from build123d import *

# Parameters (mm, degrees)
BOSS_EXTRUDE1_DEPTH      = 2
BOSS_EXTRUDE1_DEPTH_BACK = 0.2
SKETCH1_W                = 4.602701487
SKETCH1_H                = 5.995472756
SKETCH1_W_2              = 1.15
SKETCH1_H_2              = 4.4
BOSS_EXTRUDE2_REACH      = 8.943
SKETCH4_W                = 1.15
SKETCH4_H                = 4.5
CUT_EXTRUDE2_DEPTH       = 2.2
FILLET1_R                = 0.5
FILLET2_R                = 0.3


with BuildPart() as part:
    # Sketch1 → Boss-Extrude1 (new, two sides: drawn at the far end of the back side and taken through both)
    with BuildSketch(Plane(origin=(0, 0, 0), x_dir=(1, 0, 0), z_dir=(0, 1, 0)).offset(-BOSS_EXTRUDE1_DEPTH_BACK)):
        with Locations((0.573649256, 2.197554863)):
            Rectangle(SKETCH1_W, SKETCH1_H)
        with Locations((0.575, 2.2)):
            Rectangle(SKETCH1_W_2, SKETCH1_H_2, mode=Mode.SUBTRACT)
    extrude(amount=BOSS_EXTRUDE1_DEPTH + BOSS_EXTRUDE1_DEPTH_BACK)

    # Boss-Extrude2: up to this face of the body (flat: up to its plane)
    boss_extrude2_end = Plane(part.part.faces().sort_by_distance((0.573649257, 0.9, -5.195291241))[0])
    # Sketch3 → Boss-Extrude2 (add, up to the picked face)
    with BuildSketch(Plane.XY.offset(0.800181515), mode=Mode.PRIVATE) as boss_extrude2_sk1:
        with BuildLine():
            Line((-2.24541451, 7.819063766), (-1.512315748, 7.085965005))
            ThreePointArc((-1.512315748, 7.085965005), (0.573649257, 2.05), (2.659614261, 7.085965005))
            Line((2.659614261, 7.085965005), (3.399551047, 7.82590179))
            ThreePointArc((3.399551047, 7.82590179), (0.585339186, 0.994625964), (-2.24541451, 7.819063766))
        make_face()
    boss_extrude2_tool1 = split(extrude(boss_extrude2_sk1.sketch, amount=-BOSS_EXTRUDE2_REACH, mode=Mode.PRIVATE), bisect_by=boss_extrude2_end, keep=Keep.BOTH, mode=Mode.PRIVATE)
    add(boss_extrude2_tool1.solids().sort_by(Axis((-1.953222, 7.378157, 0.800182), (0, 0, -1)))[0])

    # Sketch4 → Cut-Extrude2 (cut)
    with BuildSketch(Plane.XZ):
        with Locations((0.575, -2.2)):
            Rectangle(SKETCH4_W, SKETCH4_H)
    extrude(amount=-CUT_EXTRUDE2_DEPTH, mode=Mode.SUBTRACT)

    # Fillet1
    fillet1_edges = [part.edges().sort_by_distance(p)[0] for p in [
        (-1.727701487, -0.2, -2.197554863),
        (2.875, -0.2, -2.197554863),
    ]]
    fillet(fillet1_edges, radius=FILLET1_R)

    # Fillet2
    # the kernel refuses this fillet: 0.3 mm, written as the material it takes off along each edge
    with BuildSketch(Plane(origin=(1.15, -0.2, -4.4), x_dir=(0, 0, -1), z_dir=(-1, 0, 0)), Plane(origin=(0, -0.2, 0), x_dir=(0, 0, 1), z_dir=(1, 0, 0))) as fillet2_piece_1:
        with BuildLine():
            CenterArc((0.282842712, -0.3), FILLET2_R, 90, 70.528779366)
            Line((0, -0.2), (-0.005656854, -0.198))
            ThreePointArc((-0.005656854, -0.198), (-0.006, -0.1), (-0.006, 0))
            Line((-0.006, 0), (0, 0.006))
            Line((0, 0.006), (0.282842712, 0.006))
            Line((0.282842712, 0.006), (0.282842712, 0))
        make_face()
    extrude(amount=1.15, mode=Mode.SUBTRACT)


solid = part.part
Input: part model. Units: mm. Frame: model coordinates. A direction names the side the tool comes from. Give positions to 0.01 mm unless a question says otherwise; leave off trailing zeros. Loops run counter-clockwise (first coordinate to the right, second up) from the corner with the lowest first, then second, coordinate; pieces in that order, holes last. Notation, with made-up numbers: (47.25, -27) -> (103.25, -27) arc R26 ccw to (103.25, 1) -> close; hole circle Ø2 at (5.5, -32.5). An arc over 180 degrees is marked (long way). Answer as a JSON object with one key per item and string values. Group by question number.
Item 1: Reachability of faces 4 (the flat face through (-1.728, 1, -2)), 5 (the flat face through (2.875, 1, -2)), 6 (the flat face through (0.6, 1, -4.45)) from +Z, -Z, +X, -X, +Y, -Y: full face, straight path, thin tool, end or side. Return the list, or none.
Item 2: Line query: probe 1 along X at (y, z) = (5, -1.05); probe 2 along X at (y, z) = (3.75, -3.85); probe 3 along Y at (x, z) = (3, 0.4). Output: solid intervals per line, ascending.
Item 3: Cut plane B-B, the plane y = 5. Return the cut outline in (x, z).
Item 4: Pull-direction query (X, two-part tool) for faces 1 (the cylindrical face through (4.567, 4.699, -2.156)), 2 (the flat face through (2, 2, 0.8)), 3 (the flat face through (0.6, 1, 0.05)); classes: released by +X, released by -X, zero draft, split by the parting line, or undercut.
Item 5: Pin query (flat end, axial travel): P1, Ø2, axis at x = 0.5, z = -2.5, coming from the +Y side; P2, Ø1.6, axis at y = 1, z = -1.5, coming from the +X side; P3, Ø1.2, axis at y = 1, z = -2, coming from the +X side (3 decimals). Return the tip coordinate at first contact, or that it passes through.
Item 6: Cut plane C-C, the plane x = -2. Return the cut outline in (y, z), and give its area (3 significant figures).
Item 7: Cut plane D-D, the plane y = 1. Return the cut outline in (x, z) (3 decimals), and give its area (3 significant figures).
Checks:
{
 "1": {"face 4": "+Z, -Z, -X, -Y", "face 5": "+Z, -Z, +X, -Y", "face 6": "+Y"},
 "2": {"probe 1": "x = -3.42 to -2.38, 3.52 to 4.58", "probe 2": "x = -3.22 to -2.1, 3.25 to 4.38", "probe 3": "y = 1.81 to 3.32, 6.68 to 7.43"},
 "3": {"outline": "(-3.42, -5.2) -> (-2.38, -5.2) -> (-2.38, 0.8) -> (-3.42, 0.8) -> close; (3.52, -5.2) -> (4.58, -5.2) -> (4.58, 0.8) -> (3.52, 0.8) -> close"},
 "4": {"face 1": "released by +X", "face 2": "zero draft", "face 3": "undercut"},
 "5": {"P1": "stops at y = 2.25", "P2": "stops at x = 2.99", "P3": "stops at x = 2.875"},
 "6": {"outline": "(1.94, -5.2) -> (3.56, -5.2) -> (3.56, 0.8) -> (1.94, 0.8) -> close; (6.44, -5.2) -> (7.57, -5.2) -> (7.57, 0.8) -> (6.44, 0.8) -> close", "area": "16.5 mm²"},
 "7": {"outline": "(-1.728, -5.195) -> (2.875, -5.195) -> (2.875, 0.8) -> (-1.728, 0.8) -> close; hole (0, -4.45) -> (1.15, -4.45) -> (1.15, 0.05) -> (0, 0.05) -> close", "area": "22.4 mm²"}
}
